Autodesk Inventor part; units mm, degrees
ref_plane "Work Plane2" through (0, 13.5, 0) normal (0, 1, 0) x (-1, 0, 0)
ref_plane "Work Plane3" through (0, 0, 0) normal (0, 0, 1) x (1, 0, 0)
ref_plane "Work Plane4" through (12.5, 0, 0) normal (1, 0, 0) x (0, 1, 0)
sketch "Sketch2" plane through (0, 0, 0) normal (0, 0, 1) x (1, 0, 0)
  circle A0 centre (0, 0) radius 13.5
  dimension "d0" = 27
extrude "Base" add sketch "Sketch2" along normal blind 17.5
ref_plane "Work Plane1" through (13.5, 0, 0) normal (1, 0, 0) x (0, 1, 0)
sketch "Sketch3" plane through (13.5, 0, 0) normal (1, 0, 0) x (0, 1, 0)
  line L0 (13.5, 17.5) -> (-13.5, 17.5)
  line L1 (13.5, 0) -> (-13.5, 0)
  circle A0 centre (0, 12.5) radius 2.55
  point P0 (0, 0)
  dimension "d4" = 5.1
  dimension "d31" = 5
extrude "IR hole" cut sketch "Sketch3" against normal through all
ref_plane "Work Plane2" through (0, 13.5, 0) normal (0, 1, 0) x (-1, 0, 0)
sketch "Sketch4" plane through (0, 13.5, 0) normal (0, 1, 0) x (-1, 0, 0)
  line L0 (13.5, 17.5) -> (-13.5, 17.5) construction
  line L1 (13.5, 0) -> (-13.5, 0) construction
  circle A0 centre (0, 12.5) radius 2.55
  point P0 (0, 0)
  dimension "d7" = 5.1
  dimension "d32" = 5
extrude "LED Hole" cut sketch "Sketch4" against normal blind 13.5
sketch "Sketch7" plane through (0, 0, 0) normal (0, 0, -1) x (-1, 0, 0)
  circle A0 centre (0, 0) radius 1.25
  circle A1 centre (0, 0) radius 3.25
  dimension "d24" = 2.5
  dimension "d39" = 2
extrude "Water Tube wall" add sketch "Sketch7" along normal blind 10
fillet "Fillet1" radius 9 1 edges at (-13.5, 0, 0)
ref_plane "Work Plane3" through (0, 0, 0) normal (0, 0, 1) x (1, 0, 0)
sketch "Sketch13" plane through (0, 0, 17.5) normal (0, 0, 1) x (1, 0, 0)
  circle A0 centre (0, 0) radius 1.25
  circle A1 centre (0, 0) radius 9
  circle A2 centre (0, 0) radius 13.5
  line L0 (-9, 0) -> (9, 0)
  point P0 (-1.25, 0)
  point P1 (1.25, 0)
  dimension "d40" = 4.5
  dimension "d66" = 18
revolve "Inner cut out" cut sketch "Sketch13" angle 360 about axis through (-9, 0, 17.5) along (1, 0, 0) picked at (-6.3174, 0.8177) contours A0 L0 A1
sketch "Sketch14" plane through (0, 0, 17.5) normal (0, 0, 1) x (1, 0, 0)
  circle A0 centre (0, 11.1) radius 1.25
  line L0 (-18.9, 13.5) -> (18.9, 13.5) construction
  circle A1 centre (0, 0) radius 13.5 construction
  line L1 (0, 13.5) -> (0, 9) construction
  circle A2 centre (0, 0) radius 9 construction
  circle A3 centre (-9.6129, -5.55) radius 1.25
  circle A4 centre (9.6129, -5.55) radius 1.25
  circle A5 centre (0, 0) radius 11.1 construction
  dimension "d67" = 22.2
  dimension "d42" = 2.5
  dimension "d43" = 2.4
  dimension "d44" = 4.5
  dimension "d47" = 360
extrude "Mount screw holes" cut sketch "Sketch14" against normal blind 5
ref_plane "Work Plane4" through (12.5, 0, 0) normal (1, 0, 0) x (0, 1, 0)
sketch "Sketch15" plane through (12.5, 0, 0) normal (1, 0, 0) x (0, 1, 0)
  circle A0 centre (0, 12.5) radius 2.55
  line L0 (13.5, 17.5) -> (-13.5, 17.5)
  line L1 (-3.3, 9.2) -> (3.3, 9.2)
  line L2 (3.3, 9.2) -> (3.3, 15.8)
  line L3 (3.3, 15.8) -> (-3.3, 15.8)
  line L4 (-3.3, 15.8) -> (-3.3, 9.2)
  line L5 (-3.3, 9.2) -> (3.3, 15.8) construction
  line L6 (3.3, 9.2) -> (-3.3, 15.8) construction
  point P0 (0, 0)
  dimension "d52" = 5
  dimension "d53" = 5.1
  dimension "d54" = 6.6
  dimension "d55" = 6.6
extrude "Hole wall" add sketch "Sketch15" along normal blind 2.25
pattern_circular "Circular Pattern1" count 3 over 180 about axis through (0, 0, 0) along (0, 0, 1) of "Hole wall"
sketch "Sketch17" plane through (0, 0, 0) normal (0, 0, -1) x (-1, 0, 0)
  circle A0 centre (0, 0) radius 1.25
  circle A1 centre (0, 0) radius 1.1
  dimension "d68" = 2.5
extrude "Extrusion12" cut sketch "Sketch17" against normal blind 20 contours A0 | A1
equation "\"d8\" = 0.5 * d0"
equation "\"d52\" = d31"
equation "\"d53\" = d4"
equation "\"d55\" = d54"
properties part number "Large_mouse_poke" material "ABS Plastic"
Design review of the part built by this model. Coordinates are the model's own, in mm. A direction names the side the tool comes from. Give positions to 0.01 mm unless a question says otherwise; leave off trailing zeros. Write each loop counter-clockwise with the first axis right and the second up, starting at its lowest first coordinate (ties: lowest second). Pieces come first, ordered by that corner, then holes.
(1) Tool access review of faces 1 (the face through (-3.3, 14, 12)), 2 (the face through (-8.46, -6.03, 15.04)), 3 (the face through (14, 3.3, 12)): name each direction out of +Z, -Z, +X, -X, +Y, -Y from which nothing blocks a thin tool from reaching the whole face with its end or side.
Checked values:
face 1: +Z, -Z, -X, +Y
face 2: +Z
face 3: +Z, -Z, +X, +Y
(2) Add section B-B (y = 0). Give the number of separate pieces and of enclosed holes in the cut face, and give its area (3 significant figures).
Checked values:
separate pieces: 4
enclosed holes: 0
area: 269 mm2
(3) Mouldability with a two-part tool opening along Y and no side actions: class faces 4 (the face through (14, -3.3, 13)), 5 (the face through (-1.4, 0.05, -10)), 6 (the face through (-10, -6, 12.5)) as +Y half, -Y half, draft (parallel to the pull), parting line (faces both ways), or undercut.
Checked values:
face 4: -Y half
face 5: draft
face 6: undercut
(4) Add section A-A (z = -6.75). Give the boundary of the cut face in (x, y), and give its area (3 significant figures).
Checked values:
outline: circle Ø6.5 at (0, 0); hole circle Ø2.5 at (0, 0)
area: 28.3 mm2
(5) Wall thickness on line 1 along Y through (x, z) = (0, -5.25); line 2 along Y through (x, z) = (-8.75, 12.75); line 3 along Y through (x, z) = (7.75, 12.5): over which ranges is each line inside the solid? List them lowest first.
Checked values:
line 1: y = -3.25 to -1.25, 1.25 to 3.25
line 2: y = -10.28 to -6.45, -4.65 to -2.54, 2.54 to 10.28
line 3: y = -11.05 to -2.55, 2.55 to 11.05
(6) Clearance check with flat-ended pins moving along their axes: pin 1 Ø6 at (x, y) = (4, -0.5) entering from +Z; pin 2 Ø8 at (y, z) = (3.5, 9.5) entering from +X; pin 3 Ø0.8 at (x, y) = (-0.5, 14) entering from -Z; pin 4 Ø6 at (x, y) = (6, -6.5) entering from -Z. State where each tip first meets the part, or that it passes through.
Checked values:
pin 1: stops at z = 11.57
pin 2: stops at x = 14.75
pin 3: stops at z = 9.2
pin 4: stops at z = 0.1
